For this review, use the dimensioned drawing (mm, ordinates from the lowest corner) and the shaded views. A direction names the side the tool comes from. Give positions to 0.01 mm unless a question says otherwise; leave off trailing zeros. Loops run counter-clockwise (first coordinate to the right, second up) from the corner with the lowest first, then second, coordinate; pieces in that order, holes last. Notation, with made-up numbers: (26, -19) - (30, -19) arc R11 cw to (30, -11) - close; hole circle Ø9 at (79.5, 80.25). An arc over 180 degrees is marked (long way). Write each question's results on one line, items separated by ' | '.
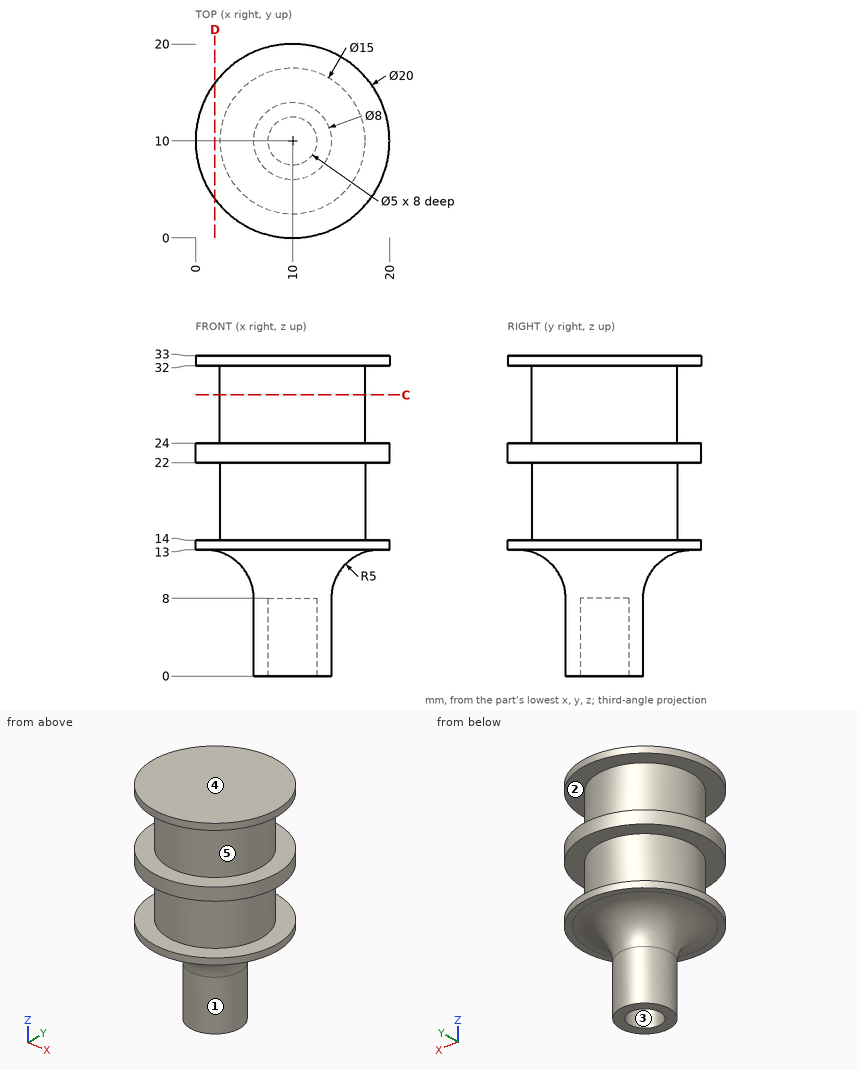
Item 1: Draft analysis for pull direction X (two halves, no side actions). For the marked faces 1, 2 and 3, state which applies: +X half, -X half, draft (parallel to the pull), parting line (faces both ways), or undercut.
Output values:
face 1: parting line | face 2: draft | face 3: undercut
Item 2: Clearance check with flat-ended pins moving along their axes: P1, Ø1, axis at x = 17.5, y = 11, coming from the -Z side; P2, Ø12, axis at y = 10, z = 3.5, coming from the +X side; P3, Ø1, axis at y = 16.5, z = 28, coming from the +X side. State where each tip first meets the part, or that it passes through.
Output values:
P1: stops at z = 12.61 | P2: stops at x = 14.23 | P3: stops at x = 14.5
Item 3: We need section D-D on x = 2. Give the number of separate pieces and of enclosed holes in the cut face, then the cut area to 3 significant figures.
Output values:
separate pieces: 3 | enclosed holes: 0 | area: 48.4 mm²
Item 4: Tool access review of the marked faces 4 and 5: name each direction out of +Z, -Z, +X, -X, +Y, -Y from which nothing blocks a thin tool from reaching the whole face with its end or side.
Output values:
face 4: +Z, +X, -X, +Y, -Y | face 5: none
Item 5: We need section C-C on z = 29. Give the boundary of the cut face in (x, y), then the cut area to 3 significant figures.
Output values:
outline: circle Ø15 at (10, 10) | area: 177 mm²
Item 6: Wall thickness on probe 1 along Y at (x, z) = (10, 3); probe 2 along Z at (x, y) = (2.25, 6.5); probe 3 along Z at (x, y) = (13.5, 2.75): over which ranges is each line inside the solid? List them lowest first.
Output values:
probe 1: y = 6 to 7.5, 12.5 to 14 | probe 2: z = 12.98 to 14, 22 to 24, 32 to 33 | probe 3: z = 12.91 to 14, 22 to 24, 32 to 33
